Geometry: final body of the model. Coordinates: model frame, mm. Face numbers are marked on the shaded views. Give positions to 0.01 mm unless a question says otherwise; leave off trailing zeros. Order: outer loops, then holes, each group sorted by start corner. A loop starts at its lowest first (then second) coordinate and runs counter-clockwise, first axis right, second up. Notation, with made-up numbers: (76.25, 81) - (91.25, 81) arc R20 ccw to (91.25, 93) - close; hole circle Ø7 at (34.25, 21.5). An arc over 180 degrees is marked (long way). Put each result on its own line as item: value. Start each with the question number.
1. Ray query, line 1 along Z through (x, y) = (-4.5, 127); line 2 along X through (y, z) = (207.5, -7). Return the intervals inside material, ascending. Write a range as from..to.
2. First-contact query: P1, Ø4, axis at x = -0.5, z = -5, coming from the +Y side. Flat tip, straight axial feed; report the tip coordinate or a pass-through.
3. Section A-A on y = 75. Return the cut outline in (x, z), plus the area to 3 significant figures.
4. Section C-C on y = 29. Return the cut outline in (x, z), plus the area to 3 significant figures.
5. Mould query, pull axis Z, two halves, no side actions, for the marked faces 1, 2 and 3. Classes: pulls with the +Z half, pulls with the -Z half, needs draft (parallel to the pull), parting line crosses it, or undercut.
6. Section B-B on z = 4.5. Return the cut outline in (x, y).
from build123d import *

# Parameters (mm, degrees)
SKETCH_1_W          = 15
SKETCH_1_H          = 15
SKETCH_1_W_2        = 13
SKETCH_1_H_2        = 13
EXTRUDE_1_DEPTH     = 225
SKETCH_2_R          = 1.5
SKETCH_2_R_2        = 2
CUT_EXTRUDE_1_DEPTH = 226.624134347
SKETCH_3_R          = 1.5
CUT_EXTRUDE_2_DEPTH = 226.624134347


with BuildPart() as part:
    # 草图1 → 凸台-拉伸1 (new body)
    with BuildSketch(Plane(origin=(0, 0, 0), x_dir=(1, 0, 0), z_dir=(0, 1, 0))):
        Rectangle(SKETCH_1_W, SKETCH_1_H)
        Rectangle(SKETCH_1_W_2, SKETCH_1_H_2, mode=Mode.SUBTRACT)
    extrude(amount=EXTRUDE_1_DEPTH)

    # 草图2 → 切除-拉伸1 (cut, through all)
    with BuildSketch(Plane.XY.offset(7.5)):
        with Locations((0, 207.5)):
            Circle(SKETCH_2_R)
        with Locations((0, 187.5)):
            Circle(SKETCH_2_R)
        with Locations((0, 75)):
            Circle(SKETCH_2_R_2)
        Polygon((7.5, 225), (-7.5, 225), (-7.5, 210), align=None)
    extrude(amount=-CUT_EXTRUDE_1_DEPTH, mode=Mode.SUBTRACT)

    # 草图3 → 切除-拉伸2 (cut, through all)
    with BuildSketch(Plane(origin=(7.5, 0, 0), x_dir=(0, 0, -1), z_dir=(1, 0, 0))):
        with Locations((0, 5)):
            Circle(SKETCH_3_R)
        with Locations((0, 20)):
            Circle(SKETCH_3_R)
        with Locations((0, 127.5)):
            Circle(SKETCH_3_R)
        with Locations((0, 147.5)):
            Circle(SKETCH_3_R)
        with Locations((0, 107.5)):
            Circle(SKETCH_3_R)
    extrude(amount=-CUT_EXTRUDE_2_DEPTH, mode=Mode.SUBTRACT)


solid = part.part
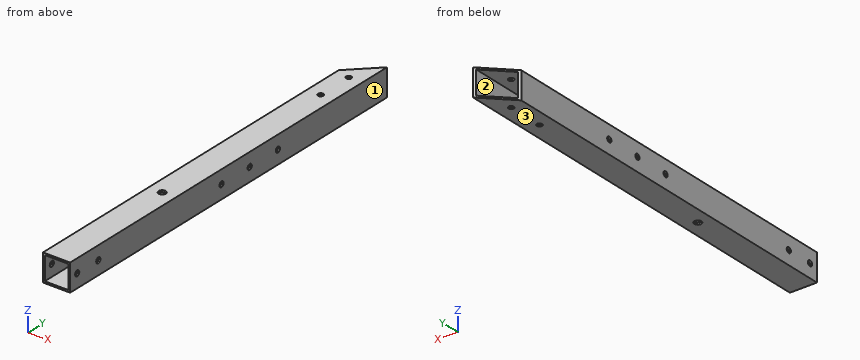
Resolved:
1. line 1: -7.5..-6.5, 6.5..7.5
1. line 2: -7.5..-1.5, 1.5..7.5
2. P1: y = 218.32
3. outline: (-7.5, -7.5) - (-2, -7.5) - (-2, -6.5) - (-6.5, -6.5) - (-6.5, 6.5) - (-2, 6.5) - (-2, 7.5) - (-7.5, 7.5) - close; (2, -7.5) - (7.5, -7.5) - (7.5, 7.5) - (2, 7.5) - (2, 6.5) - (6.5, 6.5) - (6.5, -6.5) - (2, -6.5) - close
3. area: 48.0 mm^2
4. outline: (-7.5, -7.5) - (7.5, -7.5) - (7.5, 7.5) - (-7.5, 7.5) - close; hole (-6.5, -6.5) - (6.5, -6.5) - (6.5, 6.5) - (-6.5, 6.5) - close
4. area: 56.0 mm^2
5. face 1: needs draft
5. face 2: undercut
5. face 3: pulls with the -Z half
6. outline: (-7.5, 0) - (-6.5, 0) - (-6.5, 211) - (-7.5, 210) - close; (6.5, 0) - (7.5, 0) - (7.5, 225) - (6.5, 224) - close
